Verification items for the finished model (mm, model axes). Face numbers are marked on the shaded views. Give positions to 0.01 mm unless a question says otherwise; leave off trailing zeros. Loops run counter-clockwise (first coordinate to the right, second up) from the corner with the lowest first, then second, coordinate; pieces in that order, holes last. Notation, with made-up numbers: M -18.75,86 L 14.25,86 A23 ccw 14.25,101 Z; hole C 52.5,-6.75 d1. An arc over 180 degrees is marked long. Answer in a Markdown table with one row per item.
```python
from build123d import *

# Parameters (mm, degrees)
SKETCH_1_W          = 10
SKETCH_1_H          = 5
SKETCH_1_R          = 1.55
EXTRUDE_1_DEPTH     = 1.9
SKETCH_2_W          = 30
SKETCH_2_H          = 10
EXTRUDE_2_DEPTH     = 10
SKETCH_3_R          = 4
CUT_EXTRUDE_1_DEPTH = 10


with BuildPart() as part:
    # 草图1 → 凸台-拉伸1 (new body)
    with BuildSketch(Plane(origin=(0, 0, 0), x_dir=(1, 0, 0), z_dir=(0, 1, 0))):
        with Locations((5, 2.5)):
            Rectangle(SKETCH_1_W, SKETCH_1_H)
        with Locations(Location((7, 2.5, 0), (0, 0, 90))):
            Circle(SKETCH_1_R, mode=Mode.SUBTRACT)
    extrude(amount=EXTRUDE_1_DEPTH)

    # 草图2 → 凸台-拉伸2 (add)
    with BuildSketch(Plane.ZY):
        with Locations((-2.5, 0.95)):
            Rectangle(SKETCH_2_W, SKETCH_2_H)
    extrude(amount=EXTRUDE_2_DEPTH)

    # 草图3 → 切除-拉伸1 (cut)
    with BuildSketch(Plane(origin=(0, 5.95, 0), x_dir=(1, 0, 0), z_dir=(0, 1, 0))):
        with Locations((-5, 16.3)):
            Circle(SKETCH_3_R)
        with Locations((-5, -11.3)):
            Circle(SKETCH_3_R)
    extrude(amount=-CUT_EXTRUDE_1_DEPTH, mode=Mode.SUBTRACT)


solid = part.part
```
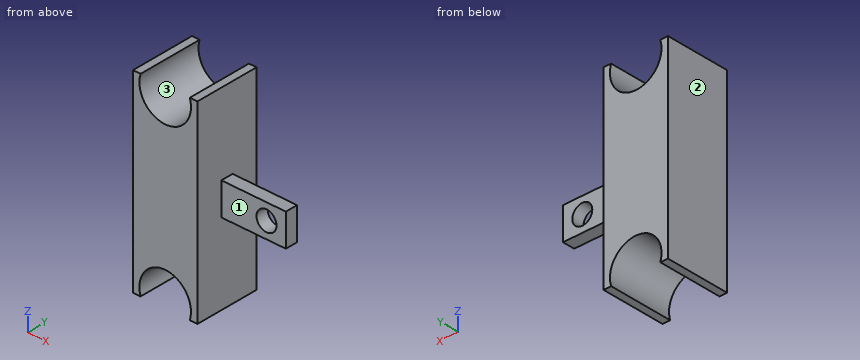
Item 1: Sectioned sample at D-D (z = -2.5). Record the cut outline in (x, y), and give its area (3 significant figures).
Reported:
| item | result |
|---|---|
| outline | M -10,-4.05 L 0,-4.05 L 0,0 L 5.45,0 L 5.45,1.9 L 0,1.9 L 0,5.95 L -10,5.95 Z; M 8.55,0 L 10,0 L 10,1.9 L 8.55,1.9 Z |
| area | 113 mm^2 |
Item 2: Go/stop test with flat-tipped pins: pin 1 (1 mm diameter, centred on y = -0.5, z = 7.5, fed in from +X); pin 2 (1 mm diameter, centred on x = 5, y = 1, fed in from -Z); pin 3 (1 mm diameter, centred on x = 5.5, y = 1, fed in from +Z); pin 4 (7 mm diameter, centred on x = -5, z = 11.3, fed in from -Y). Record where each tip stops, or that it passes through.
Reported:
| item | result |
|---|---|
| pin 1 | stops at x = 0 |
| pin 2 | stops at z = -5 |
| pin 3 | stops at z = 0 |
| pin 4 | passes through |
Item 3: Release check for a two-part mould opening along X. For the marked faces 1, 2 and 3 record: released by +X, released by -X, zero draft, split by the parting line, or undercut.
Reported:
| item | result |
|---|---|
| face 1 | zero draft |
| face 2 | released by -X |
| face 3 | undercut |
Item 4: Sectioned sample at C-C (y = -2.25). Record the cut outline in (x, z).
Reported:
| item | result |
|---|---|
| outline | M -10,-17.5 L -8.82,-17.5 A4 cw long -1.18,-17.5 L 0,-17.5 L 0,12.5 L -1.18,12.5 A4 cw long -8.82,12.5 L -10,12.5 Z |
Item 5: Scan lines: L1, parallel to X at y = 0.75, z = 11.3; L2, parallel to Z at x = 7, y = 0.45; L3, parallel to X at y = 1.1, z = -2.5. Record each from-to range of solid material in increasing order. Write a range as [from, to].
Reported:
| item | result |
|---|---|
| L1 | x = [-10, -9], [-1, 0] |
| L2 | z = [-5, -4.05], [-0.95, 0] |
| L3 | x = [-10, 5.45], [8.55, 10] |
Item 6: Sectioned sample at A-A (x = 7). Record the cut outline in (y, z).
Reported:
| item | result |
|---|---|
| outline | M 0,-5 L 1.9,-5 L 1.9,-4.05 L 0,-4.05 Z; M 0,-0.95 L 1.9,-0.95 L 1.9,0 L 0,0 Z |
Item 7: Sectioned sample at B-B (z = -16.3). Record the cut outline in (x, y).
Reported:
| item | result |
|---|---|
| outline | M -10,-4.05 L -9,-4.05 L -9,5.95 L -10,5.95 Z; M -1,-4.05 L 0,-4.05 L 0,5.95 L -1,5.95 Z |
